Here's how the part is built. I have some questions about the finished solid (model axes, mm). Face numbers are marked on the shaded views. Round coordinates to 2 decimals unless told otherwise and drop trailing zeros. Order: outer loops, then holes, each group sorted by start corner. A loop starts at its lowest first (then second) coordinate and runs counter-clockwise, first axis right, second up. Notation, with made-up numbers: (-17, 81) - (17, 81) arc R13 ccw to (17, 88) - close; hole circle Ø9 at (-38.75, 24). An arc over 180 degrees is marked (long way). One line per item, written item: value.
from build123d import *

# Parameters (mm, degrees)
F0_R     = 8.5
F1_DEPTH = 50
F2_DEPTH = 1.25


with BuildPart() as f1:
    # F0 (on Top) → F1 (new body)
    with BuildSketch(Plane.XY):
        with BuildLine():
            ThreePointArc((9.2870878105, -2), (9.4466219941, -1.0056504861), (9.5, 0))
            ThreePointArc((9.5, 0), (9.4466219941, 1.0056504861), (9.2870878105, 2))
            Line((9.2870878105, 2), (8.8004730493, 2))
            Line((8.8004730493, 2), (8.8004730493, -2))
            Line((8.8004730493, -2), (9.2870878105, -2))
        make_face()
        with BuildLine():
            ThreePointArc((9.2870878105, 2), (9.4466219941, 1.0056504861), (9.5, 0))
            ThreePointArc((9.5, 0), (9.4466219941, -1.0056504861), (9.2870878105, -2))
            Line((9.2870878105, -2), (10.1995269507, -2))
            Line((10.1995269507, -2), (10.1995269507, 2))
            Line((10.1995269507, 2), (9.2870878105, 2))
        make_face()
        with BuildLine():
            Line((8.8004730493, 2), (9.2870878105, 2))
            ThreePointArc((9.2870878105, 2), (-9.5, 0), (9.2870878105, -2))
            Line((9.2870878105, -2), (8.8004730493, -2))
            Line((8.8004730493, -2), (8.8004730493, 2))
        make_face()
        Circle(F0_R, mode=Mode.SUBTRACT)
    extrude(amount=F1_DEPTH)

    # F0 (on Top) → F2 (join)
    with BuildSketch(Plane.XY):
        with BuildLine():
            Line((8.8004730493, 2), (9.2870878105, 2))
            ThreePointArc((9.2870878105, 2), (-9.5, 0), (9.2870878105, -2))
            Line((9.2870878105, -2), (8.8004730493, -2))
            Line((8.8004730493, -2), (8.8004730493, 2))
        make_face()
        Circle(F0_R, mode=Mode.SUBTRACT)
        Circle(F0_R)
        with BuildLine():
            ThreePointArc((9.2870878105, 2), (9.4466219941, 1.0056504861), (9.5, 0))
            ThreePointArc((9.5, 0), (9.4466219941, -1.0056504861), (9.2870878105, -2))
            Line((9.2870878105, -2), (10.1995269507, -2))
            Line((10.1995269507, -2), (10.1995269507, 2))
            Line((10.1995269507, 2), (9.2870878105, 2))
        make_face()
        with BuildLine():
            ThreePointArc((9.2870878105, -2), (9.4466219941, -1.0056504861), (9.5, 0))
            ThreePointArc((9.5, 0), (9.4466219941, 1.0056504861), (9.2870878105, 2))
            Line((9.2870878105, 2), (8.8004730493, 2))
            Line((8.8004730493, 2), (8.8004730493, -2))
            Line((8.8004730493, -2), (9.2870878105, -2))
        make_face()
    extrude(amount=-F2_DEPTH)


solid = f1.part
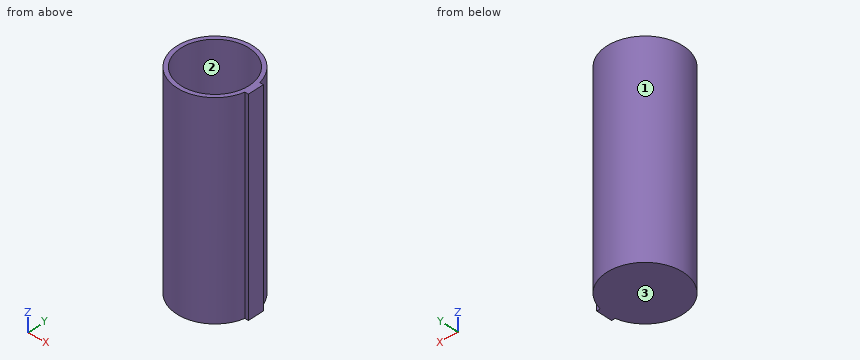
Q1. If I drill on line 1 along Y through (x, z) = (0, 11); line 2 along Z through (x, y) = (6.75, -3); line 3 along Y through (x, z) = (5.5, 8), over which ranges is the centre line in solid material (lowest first)?
Results list:
line 1: -9.5 to -8.5, 8.5 to 9.5
line 2: -1.25 to 0
line 3: -7.75 to -6.48, 6.48 to 7.75
Q2. If we section it at B-B, the plane y = 0: Please give me the cut outline in (x, z).
Results list:
outline: (-9.5, -1.25) - (10.2, -1.25) - (10.2, 50) - (8.5, 50) - (8.5, 0) - (-8.5, 0) - (-8.5, 50) - (-9.5, 50) - close
Q3. We'd pull the mould along Y, two halves only. Please class the marked faces 1, 2 and 3: released by +Y, released by -Y, zero draft, split by the parting line, or undercut.
Results list:
face 1: split by the parting line
face 2: undercut
face 3: zero draft
Q4. If we section it at A-A, the plane z = 12.5: Please give me the cut outline in (x, y).
Results list:
outline: (9.29, -2) - (10.2, -2) - (10.2, 2) - (9.29, 2) arc R9.5 ccw (long way) to start; hole circle Ø17 at (0, 0)
Q5. If we section it at C-C, the plane x = 0: Please give me the cut outline in (y, z).
Results list:
outline: (-9.5, -1.25) - (9.5, -1.25) - (9.5, 50) - (8.5, 50) - (8.5, 0) - (-8.5, 0) - (-8.5, 50) - (-9.5, 50) - close
Q6. Will these pins go through, and if not, where does the flat tip stop? pin 1 (4 mm diameter, centred on y = -7, z = 30.5, fed in from +X); pin 2 (5 mm diameter, centred on x = 3.5, z = 12.5, fed in from -Y); pin 3 (6 mm diameter, centred on y = 6.5, z = 23, fed in from -X).
Results list:
pin 1: x = 8.08
pin 2: y = -9.45
pin 3: x = -8.83
